```python
from build123d import *

# Parameters (mm, degrees)
F0_R     = 914.4
F1_DEPTH = 25.4
F2_W     = 50.8
F2_H     = 50.8
F3_DEPTH = 762


with BuildPart() as f1:
    # F0 (on Top) → F1 (new body)
    with BuildSketch(Plane.XY):
        Circle(F0_R)
    extrude(amount=-F1_DEPTH)

    # F2 (on Top) → F3 (join)
    with BuildSketch(Plane.XY):
        with Locations((482.6, -482.6)):
            Rectangle(F2_W, F2_H)
        with Locations((482.6, 482.6)):
            Rectangle(F2_W, F2_H)
        with Locations((-482.6, 482.6)):
            Rectangle(F2_W, F2_H)
        with Locations((-482.6, -482.6)):
            Rectangle(F2_W, F2_H)
    extrude(amount=-F3_DEPTH)


solid = f1.part
```
Geometry check sheet. Reference: the model listing, model coordinates, mm. A direction names the side the tool comes from. Coordinates: 2 decimals unless noted, no trailing zeros. Order: outer loops, then holes, each group sorted by start corner. A loop starts at its lowest first (then second) coordinate and runs counter-clockwise, first axis right, second up. Notation, with made-up numbers: (-3, 52) - (1, 52) arc R8 cw to (1, 64) - close; hole circle Ø6 at (59.25, 42). An arc over 180 degrees is marked (long way). Answer in a Markdown table with one row per item. Add a question column.
1. Draft check along Y on faces 1 (the face through (508, 482, -389)), 2 (the face through (-483, 457.2, -389)), 3 (the face through (482, -508, -389)), 4 (the face through (-483, 508, -389)). Enter one of: +Y half, -Y half, draft (parallel to the pull), parting line (faces both ways), or undercut.
2. Section check A-A (z = -673). Enter the section's corners in (x, y).
3. Section check B-B (x = 0). Enter the section's corners in (y, z).
4. Access from +Z, -Z, +X, -X, +Y, -Y to the whole of each face (thin tool, end or side, straight path). Record for faces 5 (the face through (482, 457.2, -389)), 6 (the face through (-457.2, 482, -389)), 7 (the face through (482, 508, -389)).
5. Material ranges on L1, parallel to Z at x = -404, y = 820; L2, parallel to X at y = 464.5, z = -720, recorded low to high. Write a range as [from, to].
6. Gauge pin test, flat ends, axial feed: pin 1 Ø8 at (x, y) = (690.5, -507.5) entering from -Z; pin 2 Ø15 at (x, z) = (490, -285) entering from +Y; pin 3 Ø15 at (y, z) = (-482, -241) entering from -X. Record the tip position at first contact, or that the pin passes through.
Data:
| question | item | result |
|---|---|---|
| 1 | face 1 | draft |
| 1 | face 2 | undercut |
| 1 | face 3 | -Y half |
| 1 | face 4 | +Y half |
| 2 | outline | (-508, -508) - (-457.2, -508) - (-457.2, -457.2) - (-508, -457.2) - close; (-508, 457.2) - (-457.2, 457.2) - (-457.2, 508) - (-508, 508) - close; (457.2, -508) - (508, -508) - (508, -457.2) - (457.2, -457.2) - close; (457.2, 457.2) - (508, 457.2) - (508, 508) - (457.2, 508) - close |
| 3 | outline | (-914.4, -25.4) - (914.4, -25.4) - (914.4, 0) - (-914.4, 0) - close |
| 4 | face 5 | -Z, +X, -X |
| 4 | face 6 | -Z, +Y, -Y |
| 4 | face 7 | -Z, +X, -X, +Y |
| 5 | L1 | z = [-25.4, 0] |
| 5 | L2 | x = [-508, -457.2], [457.2, 508] |
| 6 | pin 1 | stops at z = -25.4 |
| 6 | pin 2 | stops at y = 508 |
| 6 | pin 3 | stops at x = -508 |
